from build123d import *

# Parameters (mm, degrees)
ESBO_O1_W                = 390
ESBO_O1_H                = 95
RESSALTO_EXTRUS_O1_DEPTH = 9.525
ESBO_O3_R                = 16
CORTE_EXTRUS_O2_DEPTH    = 9.525
ESBO_O17_R               = 2.78
CORTE_EXTRUS_O12_DEPTH   = 9.525
ESBO_O18_R               = 2
CORTE_EXTRUS_O13_DEPTH   = 20
CORTE_EXTRUS_O14_START   = -20
ESBO_O19_R               = 2
CORTE_EXTRUS_O14_DEPTH   = 20


with BuildPart() as part:
    # Esboço1 → Ressalto-extrusão1 (new body)
    with BuildSketch(Plane.XY):
        Rectangle(ESBO_O1_W, ESBO_O1_H)
    extrude(amount=RESSALTO_EXTRUS_O1_DEPTH)

    # Esboço3 → Corte-extrusão2 (cut)
    with BuildSketch(Plane.XY.offset(9.525)):
        with Locations((-0.011971039, -8.12)):
            Circle(ESBO_O3_R)
    extrude(amount=-CORTE_EXTRUS_O2_DEPTH, mode=Mode.SUBTRACT)

    # Esboço17 → Corte-extrusão12 (cut)
    with BuildSketch(Plane(origin=(0, 0, 0), x_dir=(-1, 0, 0), z_dir=(0, 0, -1))):
        with Locations((23.311971039, -31.42)):
            Circle(ESBO_O17_R)
        with Locations((-23.288028961, -31.42)):
            Circle(ESBO_O17_R)
        with Locations((23.311971039, 15.18)):
            Circle(ESBO_O17_R)
        with Locations((-23.288028961, 15.18)):
            Circle(ESBO_O17_R)
    extrude(amount=-CORTE_EXTRUS_O12_DEPTH, mode=Mode.SUBTRACT)

    # Esboço18 → Corte-extrusão13 (cut)
    with BuildSketch(Plane(origin=(0, 47.5, 0), x_dir=(-1, 0, 0), z_dir=(0, 1, 0))):
        with Locations(Location((-175, 4.7625, 0), (0, 0, 90))):
            Circle(ESBO_O18_R)
        with Locations(Location((-85, 4.7625, 0), (0, 0, 90))):
            Circle(ESBO_O18_R)
        with Locations(Location((0, 4.7625, 0), (0, 0, 90))):
            Circle(ESBO_O18_R)
        with Locations(Location((175, 4.7625, 0), (0, 0, 270))):
            Circle(ESBO_O18_R)
        with Locations(Location((85, 4.7625, 0), (0, 0, 270))):
            Circle(ESBO_O18_R)
    extrude(amount=-CORTE_EXTRUS_O13_DEPTH, mode=Mode.SUBTRACT)

    # Esboço19 → Corte-extrusão14 (cut)
    with BuildSketch(Plane.XZ.offset(47.5).offset(CORTE_EXTRUS_O14_START)):
        with Locations(Location((-115, 4.7625, 0), (0, 0, 270))):
            Circle(ESBO_O19_R)
        with Locations(Location((0, 4.7625, 0), (0, 0, 90))):
            Circle(ESBO_O19_R)
        with Locations(Location((115, 4.7625, 0), (0, 0, 270))):
            Circle(ESBO_O19_R)
    extrude(amount=CORTE_EXTRUS_O14_DEPTH, mode=Mode.SUBTRACT)


solid = part.part
Geometry: final body of the model. Coordinates: model frame, mm. Give positions to 0.01 mm unless a question says otherwise; leave off trailing zeros. Order: outer loops, then holes, each group sorted by start corner. A loop starts at its lowest first (then second) coordinate and runs counter-clockwise, first axis right, second up. Notation, with made-up numbers: (48.25, 6) - (99.25, 6) arc R21 ccw to (99.25, 38) - close; hole circle Ø2 at (48, 76). An arc over 180 degrees is marked (long way). Use CSV: the item, a comma, the result in double quotes.
1. Material intervals for line 1 along Z through (x, y) = (-175, 41.5) (1 decimal); line 2 along Y through (x, z) = (1.5, 2.75); line 3 along X through (y, z) = (-29, 8), sorted ascending. Write a range as from..to.
Answers below:
line 1,"0..2.8, 6.8..9.5"
line 2,"-47.5..-24.05, 7.81..47.5"
line 3,"-195..-24.68, -21.94..21.92, 24.66..195"
2. Contact query for flat-ended pins moving along their axis: pin 1 (5 mm diameter, centred on x = -23.31, y = -31.42, fed in from -Z) (3 decimals); pin 2 (3 mm diameter, centred on x = 115, z = 4.76, fed in from -Y). Output: stop coordinate, or through.
Answers below:
pin 1,"through"
pin 2,"y = -27.5"
3. Section query B-B (z = 4.5). Give the number of separate pieces and of enclosed holes in the cut face, plus the area to 3 significant figures.
Answers below:
separate pieces,"1"
enclosed holes,"5"
area,"35,500 mm2"
4. Section query A-A (y = 34). Output: boundary loops of the cut face in (x, z) (1 decimal), plus the area to 3 significant figures.
Answers below:
outline,"(-195, 0) - (195, 0) - (195, 9.5) - (-195, 9.5) - close; hole circle Ø4 at (-175, 4.8); hole circle Ø4 at (-85, 4.8); hole circle Ø4 at (0, 4.8); hole circle Ø4 at (85, 4.8); hole circle Ø4 at (175, 4.8)"
area,"3,650 mm2"
5. Mould query, pull axis Y, two halves, no side actions, for faces 1 (the face through (195, -1, 5)), 2 (the face through (-3, 47.5, 5)), 3 (the face through (15.25, -3.31, 4.83)). Classes: +Y half, -Y half, draft (parallel to the pull), parting line (faces both ways), or undercut.
Answers below:
face 1,"draft"
face 2,"+Y half"
face 3,"undercut"
